Here's how the part is built. I have some questions about the finished solid (model axes, mm). Coordinates: 2 decimals unless noted, no trailing zeros. Write each loop counter-clockwise with the first axis right and the second up, starting at its lowest first coordinate (ties: lowest second). Pieces come first, ordered by that corner, then holes. Notation, with made-up numbers: (12.5, 33) -> (39.5, 33) arc R21 cw to (39.5, 49) -> close; hole circle Ø1 at (3, -36). An arc over 180 degrees is marked (long way). Put each result on its own line as item: value. Start each with the question number.
Item 1: I want a section at A-A, the plane z = 1.5. List the corners of the cut face in (x, y) for me, then the cut area to 3 significant figures.
Item 2: I need wall thicknesses on line 1 (X direction, y = 16.25, z = 11.5); line 2 (Z direction, x = -144.5, y = 12); line 3 (Y direction, x = -149, z = 20). Which ranges of each line are inside material? Lowest first, please. Write a range as [from, to].
Item 3: For pin 1 (8 mm diameter, centred on y = 10.5, z = 12.5, fed in from -X); pin 2 (5 mm diameter, centred on y = 8.5, z = 4, fed in from +X); pin 3 (2 mm diameter, centred on x = -126.5, y = 13.5, fed in from +Z), each with a flat end and sliding along its axis, tell me the tip position at first contact or that it passes through.
Item 4: I want a section at B-B, the plane y = 4.75. List the corners of the cut face in (x, z) for me, then the cut area to 3 significant figures.
from build123d import *

# Parameters (mm, degrees)
SKETCH1_W           = 90
SKETCH1_H           = 50
BOSS_EXTRUDE1_DEPTH = 25
SKETCH2_RX          = 3.012998166
SKETCH2_RY          = 1.246882068
BOSS_EXTRUDE2_DEPTH = 120
SKETCH3_RX          = 3.386952559
SKETCH3_RY          = 1.327839356
BOSS_EXTRUDE3_DEPTH = 25


with BuildPart() as part:
    # Sketch1 → Boss-Extrude1 (new body)
    with BuildSketch(Plane(origin=(0, 0, 0), x_dir=(1, 0, 0), z_dir=(0, 1, 0))):
        with Locations((-42.805614477, -21.913)):
            Rectangle(SKETCH1_W, SKETCH1_H)
    extrude(amount=BOSS_EXTRUDE1_DEPTH)

    # Sketch2 → Boss-Extrude2 (add)
    with BuildSketch(Plane.ZY.offset(87.805614477)):
        with Locations((21.913, 12.5)):
            Ellipse(SKETCH2_RX, SKETCH2_RY)
    extrude(amount=BOSS_EXTRUDE2_DEPTH)

    # Sketch3 → Boss-Extrude3 (add)
    with BuildSketch(Plane(origin=(2.194385523, 0, 0), x_dir=(0, 0, -1), z_dir=(1, 0, 0))):
        with Locations((-21.913, 12.5)):
            Ellipse(SKETCH3_RX, SKETCH3_RY)
    extrude(amount=BOSS_EXTRUDE3_DEPTH)


solid = part.part
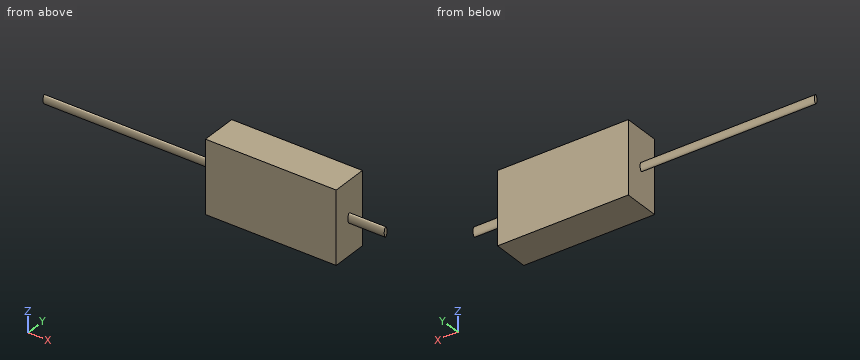
Calculated:
1. outline: (-87.81, 0) -> (2.19, 0) -> (2.19, 25) -> (-87.81, 25) -> close
1. area: 2,250 mm2
2. line 1: x = [-87.81, 2.19]
2. line 2: z = [19.15, 24.67]
2. line 3: y = [11.54, 13.46]
3. pin 1: stops at x = -87.81
3. pin 2: stops at x = 2.19
3. pin 3: stops at z = 24.93
4. outline: (-87.81, -3.09) -> (2.19, -3.09) -> (2.19, 46.91) -> (-87.81, 46.91) -> close
4. area: 4,500 mm2
